Here's how the part is built. I have some questions about the finished solid (model axes, mm). A direction names the side the tool comes from. Round coordinates to 2 decimals unless told otherwise and drop trailing zeros. Order: outer loops, then holes, each group sorted by start corner. A loop starts at its lowest first (then second) coordinate and runs counter-clockwise, first axis right, second up.
```python
from build123d import *

# Parameters (mm, degrees)
BOSS_EXTRUDE1_DEPTH = 50.8
SKETCH3_R           = 1.397
BOSS_EXTRUDE2_DEPTH = 6.35
SKETCH4_W           = 28.015
SKETCH4_H           = 25.618
CUT_EXTRUDE1_DEPTH  = 11.939


with BuildPart() as part:
    # Sketch1 → Boss-Extrude1 (new body)
    with BuildSketch(Plane.XY.offset(438.358905075)):
        with BuildLine():
            Line((42.509706517, 19.30434166), (42.509706517, 15.95534166))
            Line((42.509706517, 15.95534166), (106.009706517, 15.95534166))
            Line((106.009706517, 15.95534166), (106.009706517, 13.41534166))
            Line((106.009706517, 13.41534166), (42.509706517, 13.41534166))
            Line((42.509706517, 13.41534166), (42.509706517, 10.06634166))
            Line((42.509706517, 10.06634166), (38.725206517, 10.06634166))
            ThreePointArc((38.725206517, 10.06634166), (38.189219577, 9.8443286), (37.967206517, 9.30834166))
            Line((37.967206517, 9.30834166), (37.967206517, 5.01634166))
            Line((37.967206517, 5.01634166), (33.928999082, 5.01634166))
            ThreePointArc((33.928999082, 5.01634166), (33.3534432, 5.130826843), (32.865510483, 5.456853061))
            Line((32.865510483, 5.456853061), (29.322559963, 8.999803581))
            ThreePointArc((29.322559963, 8.999803581), (28.898807275, 9.839396326), (29.056588326, 10.766535722))
            ThreePointArc((29.056588326, 10.766535722), (29.726160528, 12.451998876), (30.017474414, 14.24204055))
            Line((30.017474414, 14.24204055), (29.707071635, 14.68534166))
            Line((29.707071635, 14.68534166), (30.017474414, 15.128642769))
            ThreePointArc((30.017474414, 15.128642769), (29.726160528, 16.918684443), (29.056588326, 18.604147597))
            ThreePointArc((29.056588326, 18.604147597), (28.898807275, 19.531286993), (29.322559963, 20.370879739))
            Line((29.322559963, 20.370879739), (32.865510483, 23.913830259))
            ThreePointArc((32.865510483, 23.913830259), (33.3534432, 24.239856477), (33.928999082, 24.35434166))
            Line((33.928999082, 24.35434166), (37.967206517, 24.35434166))
            Line((37.967206517, 24.35434166), (37.967206517, 20.06234166))
            ThreePointArc((37.967206517, 20.06234166), (38.189219577, 19.526354719), (38.725206517, 19.30434166))
            Line((38.725206517, 19.30434166), (42.509706517, 19.30434166))
        make_face()
    extrude(amount=-BOSS_EXTRUDE1_DEPTH)

    # Sketch3 → Boss-Extrude2 (add)
    with BuildSketch(Plane(origin=(0, 15.95534166, 0), x_dir=(1, 0, 0), z_dir=(0, 1, 0))):
        with Locations((65.411874918, -398.072421398)):
            Circle(SKETCH3_R)
        with Locations((95.411874918, -398.072421398)):
            Circle(SKETCH3_R)
        with Locations((95.411874918, -427.072421398)):
            Circle(SKETCH3_R)
        with Locations((65.411874918, -427.072421398)):
            Circle(SKETCH3_R)
    extrude(amount=BOSS_EXTRUDE2_DEPTH)

    # Sketch4 → Cut-Extrude1 (cut, through all)
    with BuildSketch(Plane(origin=(0, 15.95534166, 0), x_dir=(1, 0, 0), z_dir=(0, 1, 0))):
        with Locations((80.094374918, -412.572421398)):
            Rectangle(SKETCH4_W, SKETCH4_H)
    extrude(amount=-CUT_EXTRUDE1_DEPTH, mode=Mode.SUBTRACT)


solid = part.part
```
1. I need wall thicknesses on probe 1 along X at (y, z) = (22.25, 397); probe 2 along X at (y, z) = (17.5, 427); probe 3 along X at (y, z) = (14.25, 409). Which ranges of each line are inside material? Lowest first, please.
Evaluation:
probe 1: x = 31.2 to 37.97, 64.52 to 66.31, 94.52 to 96.31
probe 2: x = 29.54 to 42.51, 64.02 to 66.81, 94.02 to 96.81
probe 3: x = 30.01 to 66.09, 94.1 to 106.01
2. If we mould it in two halves opening along X, with no side actions, what happens to faces 1 (the cylindrical face through (64.3, 19.09, 398.92)), 2 (the cylindrical face through (64.016, 19.086, 427.011)), 3 (the flat face through (41, 10.066, 413)), 4 (the cylindrical face through (28.897, 19.518, 413.315))? For each: released by +X, released by -X, zero draft, split by the parting line, or undercut.
Evaluation:
face 1: undercut
face 2: undercut
face 3: zero draft
face 4: released by -X
3. If we section it at A-A, the plane z = 420.5: Write out the boundary of the cut face in (x, y), and give its area (3 significant figures).
Evaluation:
outline: (29.06, 10.77) arc R1.5 ccw to (29.32, 9) - (32.87, 5.46) arc R1.5 ccw to (33.93, 5.02) - (37.97, 5.02) - (37.97, 9.31) arc R0.76 cw to (38.73, 10.07) - (42.51, 10.07) - (42.51, 13.42) - (66.09, 13.42) - (66.09, 15.96) - (42.51, 15.96) - (42.51, 19.3) - (38.73, 19.3) arc R0.76 cw to (37.97, 20.06) - (37.97, 24.35) - (33.93, 24.35) arc R1.5 ccw to (32.87, 23.91) - (29.32, 20.37) arc R1.5 ccw to (29.06, 18.6) arc R8.38 cw to (30.02, 15.13) - (29.71, 14.69) - (30.02, 14.24) arc R8.38 cw to start; (94.1, 13.42) - (106.01, 13.42) - (106.01, 15.96) - (94.1, 15.96) - close
area: 282 mm2
4. I'm going to push flat-ended pins straight in: P1, Ø5, axis at y = 8.5, z = 410, coming from the +X side; P2, Ø3, axis at x = 66, z = 427, coming from the +Y side; P3, Ø10, axis at x = 85, y = 21.5, coming from the +Z side; P4, Ø6, axis at x = 92, z = 423, coming from the -Y side. Where does each tip first touch, or does it pass through?
Evaluation:
P1: stops at x = 42.51
P2: stops at y = 22.31
P3: passes through
P4: stops at y = 13.42
5. On a 3-axis mill with a long thin cutter (end or side, diameter ignored), from which of +Z, -Z, +X, -X, +Y, -Y can I reach the whole of each face in a straight line? I mean faces 5 (the flat face through (66.087, 15, 413)), 6 (the flat face through (106.01, 15, 413)), 7 (the cylindrical face through (95.109, 19.086, 399.436)), 8 (the flat face through (95, 22.305, 427)), 9 (the flat face through (50, 15, 438.359)). Say none if no direction works.
Evaluation:
face 5: +Y, -Y
face 6: +Z, -Z, +X, +Y, -Y
face 7: +Y
face 8: +Z, -Z, +X, +Y
face 9: +Z, +X, -X, +Y, -Y
6. If we section it at D-D, the plane y = 21.5: Write out the boundary of the cut face in (x, z).
Evaluation:
outline: (30.45, 387.56) - (37.97, 387.56) - (37.97, 438.36) - (30.45, 438.36) - close; circle Ø2.79 at (65.41, 398.07); circle Ø2.79 at (65.41, 427.07); circle Ø2.79 at (95.41, 398.07); circle Ø2.79 at (95.41, 427.07)
7. If we section it at B-B, the plane x = 74: Write out the boundary of the cut face in (y, z).
Evaluation:
outline: (13.42, 387.56) - (15.96, 387.56) - (15.96, 399.76) - (13.42, 399.76) - close; (13.42, 425.38) - (15.96, 425.38) - (15.96, 438.36) - (13.42, 438.36) - close
8. If we section it at C-C, the plane z = 432: Write out the boundary of the cut face in (x, y), and give its area (3 significant figures).
Evaluation:
outline: (29.06, 10.77) arc R1.5 ccw to (29.32, 9) - (32.87, 5.46) arc R1.5 ccw to (33.93, 5.02) - (37.97, 5.02) - (37.97, 9.31) arc R0.76 cw to (38.73, 10.07) - (42.51, 10.07) - (42.51, 13.42) - (106.01, 13.42) - (106.01, 15.96) - (42.51, 15.96) - (42.51, 19.3) - (38.73, 19.3) arc R0.76 cw to (37.97, 20.06) - (37.97, 24.35) - (33.93, 24.35) arc R1.5 ccw to (32.87, 23.91) - (29.32, 20.37) arc R1.5 ccw to (29.06, 18.6) arc R8.38 cw to (30.02, 15.13) - (29.71, 14.69) - (30.02, 14.24) arc R8.38 cw to start
area: 353 mm2
